```python
from build123d import *

# Parameters (mm, degrees)
F0_W     = 63.5
F0_H     = 38.1
F1_DEPTH = 6.35
F2_W     = 38.1
F2_H     = 25.4
F3_DEPTH = 75.1442132
F5_DEPTH = 9.144


# Not quite as in the source:
# - an extrude ends at something that could not be found from the text; its depth is read off the source's solid


with BuildPart() as f1:
    # F0 (on Top) → F1 (new body, symmetric)
    with BuildSketch(Plane.XY):
        Rectangle(F0_W, F0_H)
    extrude(amount=F1_DEPTH, both=True)

    # F2 (on face) → F3 (join, through all)
    with BuildSketch(Plane.XY.offset(6.35)):
        Rectangle(F2_W, F2_H)
    extrude(amount=F3_DEPTH)

    # F4 (on face) → F5 (join)
    with BuildSketch(Plane.XZ.offset(19.05)):
        with BuildLine():
            Line((-31.75, 6.35), (-10.2243826786, 6.35))
            ThreePointArc((-10.2243826786, 6.35), (-35.1404271759, 0), (-10.2243826786, -6.35))
            Line((-10.2243826786, -6.35), (-31.75, -6.35))
            Line((-31.75, -6.35), (-31.75, 6.35))
        make_face()
    extrude(amount=-F5_DEPTH)


solid = f1.part
```
Input: part model. Units: mm. Frame: model coordinates. A direction names the side the tool comes from. Coordinates: 2 decimals unless noted, no trailing zeros. Loops run counter-clockwise (first coordinate to the right, second up) from the corner with the lowest first, then second, coordinate; pieces in that order, holes last.
Q1. Line query: line 1 along Z through (x, y) = (-1, -17); line 2 along Y through (x, z) = (1, 66); line 3 along X through (y, z) = (3.5, 46). Output: solid intervals per line, ascending.
Results are:
line 1: z = -6.35 to 6.35
line 2: y = -12.7 to 12.7
line 3: x = -19.05 to 19.05
Q2. Set-up query: faces 1 (the flat face through (0, 12.7, 43)), 2 (the flat face through (-31.75, 4, 0)), 3 (the flat face through (0, 0, -6.35)). Return all of +Z, -Z, +X, -X, +Y, -Y with unobstructed straight access to the full face (end or side cutting, diameter ignored); none if empty.
Results are:
face 1: +Z, +X, -X, +Y
face 2: +Z, -Z, -X, +Y
face 3: -Z, +X, +Y
Q3. Section D-D, the plane x = 28. Return the cut outline in (y, z).
Results are:
outline: (-19.05, -6.35) - (19.05, -6.35) - (19.05, 6.35) - (-19.05, 6.35) - close
Q4. Contact query for flat-ended pins moving along their axis: pin 1 (12.5 mm diameter, centred on y = 2, z = 52, fed in from +X); pin 2 (5 mm diameter, centred on x = 6, y = 14, fed in from +Z); pin 3 (5 mm diameter, centred on x = 6.5, y = 0.5, fed in from -Z); pin 4 (20.5 mm diameter, centred on y = -5, z = 43.5, fed in from -X). Output: stop coordinate, or through.
Results are:
pin 1: stops at x = 19.05
pin 2: stops at z = 81.49
pin 3: stops at z = -6.35
pin 4: stops at x = -19.05
Q5. Section B-B, the plane y = -3. Return the cut outline in (x, z).
Results are:
outline: (-31.75, -6.35) - (31.75, -6.35) - (31.75, 6.35) - (19.05, 6.35) - (19.05, 81.49) - (-19.05, 81.49) - (-19.05, 6.35) - (-31.75, 6.35) - close
Q6. Section A-A, the plane x = 5.5. Return the cut outline in (y, z).
Results are:
outline: (-19.05, -6.35) - (19.05, -6.35) - (19.05, 6.35) - (12.7, 6.35) - (12.7, 81.49) - (-12.7, 81.49) - (-12.7, 6.35) - (-19.05, 6.35) - close
